from build123d import *

# Parameters (mm, degrees)
SKETCH2_W           = 20
SKETCH2_H           = 20
SKETCH2_R           = 2.1
BOSS_EXTRUDE1_DEPTH = 100
CUT_EXTRUDE1_DEPTH  = 101.995049384
FILLET1_R           = 0.5


with BuildPart() as part:
    # Sketch2 → Boss-Extrude1 (new body)
    with BuildSketch(Plane(origin=(0, 0, 0), x_dir=(1, 0, 0), z_dir=(0, 1, 0))):
        Rectangle(SKETCH2_W, SKETCH2_H)
        with Locations(Location((0, 0, 0), (0, 0, 270))):
            Circle(SKETCH2_R, mode=Mode.SUBTRACT)
    extrude(amount=-BOSS_EXTRUDE1_DEPTH)

    # Sketch3 → Cut-Extrude1 (cut, through all)
    with BuildSketch(Plane(origin=(0, 0, 0), x_dir=(1, 0, 0), z_dir=(0, 1, 0))):
        Polygon((5.5, -6.551650429), (2.848349571, -3.9), (-2.848349571, -3.9), (-5.5, -6.551650429), (-5.5, -8.2), (-3.7, -8.2), (-3.7, -8.7), (-5, -10), (5, -10), (3.7, -8.7), (3.7, -8.2), (5.5, -8.2), align=None)
        Polygon((3.9, 2.848349571), (3.9, -2.848349571), (6.551650429, -5.5), (8.2, -5.5), (8.2, -3.7), (8.7, -3.7), (10, -5), (10, 5), (8.7, 3.7), (8.2, 3.7), (8.2, 5.5), (6.551650429, 5.5), align=None)
        Polygon((-6.551650429, -5.5), (-3.9, -2.848349571), (-3.9, 2.848349571), (-6.551650429, 5.5), (-8.2, 5.5), (-8.2, 3.7), (-8.7, 3.7), (-10, 5), (-10, -5), (-8.7, -3.7), (-8.2, -3.7), (-8.2, -5.5), align=None)
        Polygon((-2.848349571, 3.9), (2.848349571, 3.9), (5.5, 6.551650429), (5.5, 8.2), (3.7, 8.2), (3.7, 8.7), (5, 10), (-5, 10), (-3.7, 8.7), (-3.7, 8.2), (-5.5, 8.2), (-5.5, 6.551650429), align=None)
    extrude(amount=-CUT_EXTRUDE1_DEPTH, mode=Mode.SUBTRACT)

    # Fillet1
    fillet1_edges = [part.edges().sort_by_distance(p)[0] for p in [
        (-10, -50, -10),
        (10, -50, -10),
        (10, -50, 10),
        (-10, -50, 10),
    ]]
    fillet(fillet1_edges, radius=FILLET1_R)


solid = part.part
Input: part model. Units: mm. Frame: model coordinates. A direction names the side the tool comes from. Coordinates: 2 decimals unless noted, no trailing zeros. Loops run counter-clockwise (first coordinate to the right, second up) from the corner with the lowest first, then second, coordinate; pieces in that order, holes last.
Q1. Material intervals for line 1 (X direction, y = -61, z = 0); line 2 (Z direction, x = -4.25, y = -67.5); line 3 (Z direction, x = -7.25, y = -58.5), sorted ascending.
Q2. Contact query for flat-ended pins moving along their axis: pin 1 (2 mm diameter, centred on x = 2.5, y = -42.5, fed in from -Z); pin 2 (1.5 mm diameter, centred on x = -4, y = -36, fed in from -Z); pin 3 (3 mm diameter, centred on x = 1, y = -44, fed in from +Z). Output: stop coordinate, or through.
Q3. Draft query along Z for faces 6 (the face through (-7, -49, 10)), 7 (the face through (5, -49, 8.2)), 8 (the face through (-0.1, 0, -2.4)). Return one class per face: +Z half, -Z half, draft (parallel to the pull), parting line (faces both ways), or undercut.
Q4. Cut plane A-A (z = 0). Output: boundary loops of the cut face in (x, y), then the cut area to 3 significant figures.
Q5. Set-up query: faces 1 (the face through (-3.9, -49, 0)), 2 (the face through (-7, -49, -10)), 3 (the face through (10, -49, 7)), 4 (the face through (3.9, -49, 0)), 5 (the face through (-4.19, -49.3, -5.24)). Return all of +Z, -Z, +X, -X, +Y, -Y with unobstructed straight access to the full face (end or side cutting, diameter ignored); none if empty.
Q6. Cut plane B-B (x = 0). Output: boundary loops of the cut face in (y, z).
Working result:
1. line 1: x = -3.9 to -2.1, 2.1 to 3.9
1. line 2: z = -9.25 to -8.2, -5.3 to -3.2, 3.2 to 5.3, 8.2 to 9.25
1. line 3: z = -10 to -5.5, 5.5 to 10
2. pin 1: stops at z = -4.55
2. pin 2: stops at z = -9.75
2. pin 3: stops at z = 3.9
3. face 6: +Z half
3. face 7: undercut
3. face 8: draft
4. outline: (-3.9, -100) - (-2.1, -100) - (-2.1, 0) - (-3.9, 0) - close; (2.1, -100) - (3.9, -100) - (3.9, 0) - (2.1, 0) - close
4. area: 360 mm2
5. face 1: -X, +Y, -Y
5. face 2: -Z, +X, -X, +Y, -Y
5. face 3: +Z, -Z, +X, +Y, -Y
5. face 4: +X, +Y, -Y
5. face 5: +Y, -Y
6. outline: (-100, -3.9) - (0, -3.9) - (0, -2.1) - (-100, -2.1) - close; (-100, 2.1) - (0, 2.1) - (0, 3.9) - (-100, 3.9) - close
